Geometry check sheet. Reference: the model listing, model coordinates, mm. Face numbers are marked on the shaded views. Coordinates: 2 decimals unless noted, no trailing zeros. Loops run counter-clockwise (first coordinate to the right, second up) from the corner with the lowest first, then second, coordinate; pieces in that order, holes last. Notation, with made-up numbers: (57, 24) -> (78, 24) arc R5 cw to (78, 32) -> close; hole circle Ø9 at (85, 53). An arc over 180 degrees is marked (long way). Answer as a JSON object with one key per item and string values.
from build123d import *

# Parameters (mm, degrees)
SKETCH1_R           = 7.62
SKETCH1_R_2         = 6.985
BOSS_EXTRUDE1_DEPTH = 76.2
SKETCH2_R           = 7.62
BOSS_EXTRUDE2_DEPTH = 1.27
SKETCH3_R           = 1.905
SKETCH3_R_2         = 1.27
BOSS_EXTRUDE3_DEPTH = 6.35
SKETCH4_R           = 1.27
CUT_EXTRUDE1_DEPTH  = 1.27


with BuildPart() as part:
    # Sketch1 → Boss-Extrude1 (new body)
    with BuildSketch(Plane.XY):
        Circle(SKETCH1_R)
        Circle(SKETCH1_R_2, mode=Mode.SUBTRACT)
    extrude(amount=BOSS_EXTRUDE1_DEPTH)

    # Sketch2 → Boss-Extrude2 (add)
    with BuildSketch(Plane(origin=(0, 0, 0), x_dir=(-1, 0, 0), z_dir=(0, 0, -1))):
        Circle(SKETCH2_R)
    extrude(amount=BOSS_EXTRUDE2_DEPTH)

    # Sketch3 → Boss-Extrude3 (add)
    with BuildSketch(Plane(origin=(0, 0, -1.27), x_dir=(-1, 0, 0), z_dir=(0, 0, -1))):
        Circle(SKETCH3_R)
        Circle(SKETCH3_R_2, mode=Mode.SUBTRACT)
    extrude(amount=BOSS_EXTRUDE3_DEPTH)

    # Sketch4 → Cut-Extrude1 (cut)
    with BuildSketch(Plane(origin=(0, 0, -1.27), x_dir=(-1, 0, 0), z_dir=(0, 0, -1))):
        Circle(SKETCH4_R)
    extrude(amount=-CUT_EXTRUDE1_DEPTH, mode=Mode.SUBTRACT)


solid = part.part
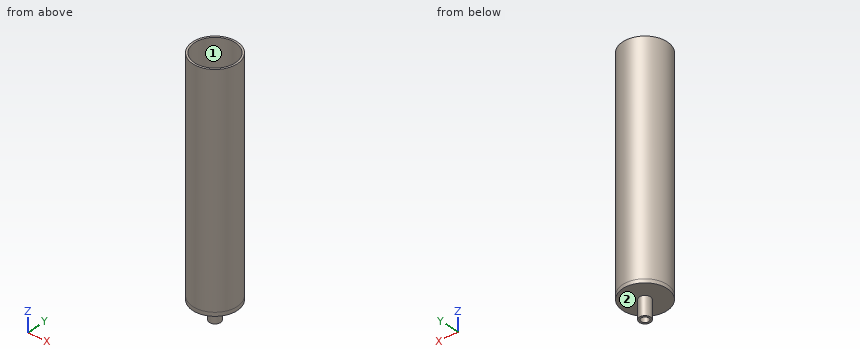
1. Mould release check, pull along Y, two halves, no side actions. Record for the marked faces 1 and 2: released by +Y, released by -Y, zero draft, split by the parting line, or undercut.
Evaluation:
{"face 1": "undercut", "face 2": "zero draft"}
2. Section check D-D, the plane y = 5.5. Record the boundary of the cut face in (x, z).
Evaluation:
{"outline": "(-5.27, -1.27) -> (5.27, -1.27) -> (5.27, 76.2) -> (4.31, 76.2) -> (4.31, 0) -> (-4.31, 0) -> (-4.31, 76.2) -> (-5.27, 76.2) -> close"}
3. Section check A-A, the plane y = 0. Record the boundary of the cut face in (x, z) (3 decimals), then the cut area to 3 significant figures.
Evaluation:
{"outline": "(-7.62, -1.27) -> (-1.905, -1.27) -> (-1.905, -7.62) -> (-1.27, -7.62) -> (-1.27, 0) -> (-6.985, 0) -> (-6.985, 76.2) -> (-7.62, 76.2) -> close; (1.27, -7.62) -> (1.905, -7.62) -> (1.905, -1.27) -> (7.62, -1.27) -> (7.62, 76.2) -> (6.985, 76.2) -> (6.985, 0) -> (1.27, 0) -> close", "area": "121 mm^2"}
4. Section check C-C, the plane z = 25. Record the boundary of the cut face in (x, y) (3 decimals), then the cut area to 3 significant figures.
Evaluation:
{"outline": "circle Ø15.24 at (0, 0); hole circle Ø13.97 at (0, 0)", "area": "29.1 mm^2"}
5. Depth check by flat-ended pin: P1, Ø1.5, axis at y = -2.5, z = 40, coming from the -X side; P2, Ø1, axis at x = -3, z = 20, coming from the +Y side; P3, Ø2, axis at x = 0, y = 0, coming from the +Z side; P4, Ø2, axis at x = 3.5, z = 3.5, coming from the -Y side. Enter the tip coordinate at first touch or a pass-through.
Evaluation:
{"P1": "stops at x = -7.42", "P2": "stops at y = 7.2", "P3": "passes through", "P4": "stops at y = -7.2"}
6. Thickness scan on probe 1 along Y at (x, z) = (0, -0.7); probe 2 along Y at (x, z) = (0, -3) (3 decimals); probe 3 along Z at (x, y) = (1.25, -4.25). Record the ranges inside material, lowest first. Write a range as from..to.
Evaluation:
{"probe 1": "y = -7.62..-1.27, 1.27..7.62", "probe 2": "y = -1.905..-1.27, 1.27..1.905", "probe 3": "z = -1.27..0"}
